Work out the finished part from the listing and answer in its coordinate system (mm). A direction names the side the tool comes from. Coordinates: 2 decimals unless noted, no trailing zeros. Write each loop counter-clockwise with the first axis right and the second up, starting at its lowest first coordinate (ties: lowest second). Pieces come first, ordered by that corner, then holes. Notation, with made-up numbers: (17, -4) - (36, -4) arc R22 cw to (36, 18) - close; hole circle Ø8 at (3.25, 13). An arc over 180 degrees is marked (long way). Use one line per item in the form item = value. Start each with the question number.
Item 1: A cutting plane is placed at B-B (x = 9.25). Write down the section's boundary in (y, z).
Item 2: A cutting plane is placed at C-C (z = -1.5). Write down the section's boundary in (x, y), then the cut area to 3 significant figures.
Item 3: Determine the mould class of faces 1 (the flat face through (0, -4, 6.5)), 2 (the cylindrical face through (2.456, -0.947, 6.007)), 3 (the cylindrical face through (5.248, -0.117, 2.049)) for opening direction Z: released by +Z, released by -Z, zero draft, split by the parting line, or undercut.
Item 4: For faces 4 (the cylindrical face through (-4.15, -0.16, 1.93)), 5 (the flat face through (7, -1, 5)), determine the directions among +Z, -Z, +X, -X, +Y, -Y from which every point of the face is accessible in a straight line to the end or side of a thin tool.
Item 5: Given pin 1 (4 mm diameter, centred on x = -4.4, y = -6.5, fed in from -Z); pin 2 (2 mm diameter, centred on y = 4, z = -6, fed in from -X); pin 3 (2.5 mm diameter, centred on x = 0, y = 0, fed in from -Z); pin 4 (1.5 mm diameter, centred on x = 2, z = -2.5, fed in from -Y), each flat-ended and moving along its own axis, determine where each tip first touches the part or whether it passes through.
Item 6: A cutting plane is placed at D-D (y = 5.75). Write down the section's boundary in (x, z), then the cut area to 3 significant figures.
Item 7: Consider probe 1 along Z at (x, y) = (2, 5.25); probe 2 along X at (y, z) = (1.5, 1.75); probe 3 along X at (y, z) = (1.75, -3.5). Determine where each line is inside the solid, lowest interval first.
Item 8: A cutting plane is placed at A-A (z = 2.5). Write down the section's boundary in (x, y), then the cut area to 3 significant figures.
Autodesk Inventor part; units mm, degrees
ref_plane "YZ Plane" through (0, 0, 0) normal (1, 0, 0) x (0, 1, 0)
ref_plane "XZ Plane" through (0, 0, 0) normal (0, 1, 0) x (-1, 0, 0)
ref_plane "XY Plane" through (0, 0, 0) normal (0, 0, 1) x (1, 0, 0)
sketch "스케치1" plane through (0, 0, 0) normal (0, 0, 1) x (1, 0, 0)
  circle A0 centre (0.5479, -1.5474) radius 5.5
  circle A1 centre (0.5479, -1.5474) radius 5
  circle A2 centre (0.5479, -1.5474) radius 4.2
  ellipse E0 centre (0.5479, -1.5474) end of major axis (-0.0909, -9.0201) minor radius 7.4992
  ellipse E1 centre (0.5479, -1.5474) end of major axis (-0.0912, -9.0201) minor radius 7.4991
  ellipse E2 centre (0.5479, -1.5474) end of major axis (1.2999, 2.3813) minor radius 3.9993 (-3.4513, -1.5143) -> (4.5471, -1.5804) ccw
  dimension "d0" = 10
  dimension "d1" = 8.4
  dimension "d24" = 11
extrude "돌출1" add sketch "스케치1" against normal blind 8 contours A1
sketch "스케치2" plane through (0.5479, -1.5474, 0) normal (0, 0, 1) x (1, 0, 0)
  circle A0 centre (0, 0) radius 4.2
  circle A1 centre (0, 0) radius 5.5
  dimension "d4" = 11
extrude "돌출2" add sketch "스케치2" along normal blind 5
sketch "스케치3" plane through (0.5479, -1.5474, 5) normal (0, 0, 1) x (1, 0, 0)
  circle A0 centre (0, 0) radius 5.5
  circle A1 centre (0, 0) radius 4.2
  circle A2 centre (0, 0) radius 10
  circle A3 centre (4.9497, -4.9497) radius 1.3
  circle A4 centre (0, 0) radius 5
  line L0 (0, 0) -> (0, -5.5) construction
  circle A5 centre (4.9497, 4.9497) radius 1.3
  circle A6 centre (-4.9497, 4.9497) radius 1.3
  circle A7 centre (-4.9497, -4.9497) radius 1.3
  dimension "d9" = 20
  dimension "d10" = 2.6
  dimension "d11" = 7
  dimension "d12" = 45
  dimension "d15" = 360
extrude "돌출3" add sketch "스케치3" along normal blind 1.5 contours A0 | A2 | A4
sketch "스케치4" plane through (0.5479, -1.5474, 6.5) normal (0, 0, 1) x (1, 0, 0)
  circle A0 centre (0, 0) radius 4.2
  circle A1 centre (0, 0) radius 2
  dimension "d17" = 4
extrude "돌출4" add sketch "스케치4" against normal blind 1
sketch "스케치5" plane through (0, 0, 0) normal (1, 0, 0) x (0, 1, 0)
  circle A0 centre (-1.5474, 2.5) radius 1.5
  line L0 (3.9526, 0) -> (-7.0474, 0)
  line L1 (3.9526, 5) -> (-7.0474, 5)
  line L2 (3.9526, 0) -> (-7.0474, 0)
  line L3 (-7.0474, 0) -> (-7.0474, 5)
  line L4 (3.9526, 0) -> (3.9526, 5)
  point P0 (0, 0)
  point P1 (-1.5474, 5)
  dimension "d20" = 3
  dimension "d21" = 2.5
extrude "돌출5" cut sketch "스케치5" along normal through all both and the other way through all contours A0
sketch "스케치6" plane through (0.5479, -1.5474, 0) normal (0, 0, -1) x (-1, 0, 0)
  circle A0 centre (0, 0) radius 5.5
  circle A1 centre (0, 0) radius 5
  point P0 (0.5479, 1.5474)
extrude "돌출6" add sketch "스케치6" along normal blind 8
properties part number "motor_clamp" material "고무, 검은색"
Answer:
q1.outline = (-6.47, 5) - (3.38, 5) - (3.38, 6.5) - (-6.47, 6.5) - close
q2.outline = circle Ø11 at (0.55, -1.55); hole circle Ø8.4 at (0.55, -1.55)
q2.area = 39.6 mm²
q3.face_1 = released by +Z
q3.face_2 = zero draft
q3.face_3 = undercut
q4.face_4 = +X, -X
q4.face_5 = -Z
q5.pin_1 = -8
q5.pin_2 = -2.55
q5.pin_3 = 5.5
q5.pin_4 = -7
q6.outline = (-6.29, 5) - (7.39, 5) - (7.39, 6.5) - (-6.29, 6.5) - close
q6.area = 20.5 mm²
q7.probe_1 = 5 to 6.5
q7.probe_2 = -4.03 to -2.34, 3.44 to 5.13
q7.probe_3 = -3.85 to -2.05, 3.15 to 4.95
q8.outline = (-4.74, -3.05) arc R5.5 ccw to (5.84, -3.05) - (4.47, -3.05) arc R4.2 cw to (-3.38, -3.05) - close; (-4.74, -0.05) - (-3.38, -0.05) arc R4.2 cw to (4.47, -0.05) - (5.84, -0.05) arc R5.5 ccw to start
q8.area = 31.7 mm²
